Verification items for the finished model (mm, model axes). A direction names the side the tool comes from. Give positions to 0.01 mm unless a question says otherwise; leave off trailing zeros. Write each loop counter-clockwise with the first axis right and the second up, starting at its lowest first coordinate (ties: lowest second). Pieces come first, ordered by that corner, then holes. Notation, with made-up numbers: (-4.75, 16) - (8.25, 16) arc R26 cw to (8.25, 44) - close; hole circle Ø8 at (21, 29). An arc over 180 degrees is marked (long way). Answer as a JSON object with one key per item and string values. Group by question number.
Item 1: Sectioned sample at C-C, the plane x = -3.5. Record the boundary of the cut face in (y, z), and give its area (3 significant figures).
Item 2: Sectioned sample at B-B, the plane x = -27. Record the boundary of the cut face in (y, z).
Item 3: Sectioned sample at A-A, the plane y = 53.5. Record the boundary of the cut face in (x, z), and give its area (3 significant figures).
Item 4: Tool access check on faces 1 (the face through (-45.11, 2, 3)), 2 (the face through (-40.462, 6, 3)), 3 (the face through (-14, 0, 3)). Record the directions out of +Z, -Z, +X, -X, +Y, -Y that give a thin tool (end or side, any length) a straight path to the whole face; none if there is none.
Item 5: Scan lines: line 1 along X through (y, z) = (8.5, 1.6); line 2 along Y through (x, z) = (-34, 0.6); line 3 along Y through (x, z) = (-21, 4.4). Record each from-to range of solid material in increasing order. Write a range as [from, to].
Item 6: Go/stop test with flat-tipped pins: pin 1 (1.4 mm diameter, centred on x = -41, z = 3, fed in from -Y); pin 2 (0.9 mm diameter, centred on x = -43.5, z = 3.5, fed in from -Y) (3 decimals). Record where each tip stops, or that it passes through.
Item 7: Draft check along Y on faces 4 (the face through (-25, 19.467, 3)), 5 (the face through (-14, 49, 0)), 6 (the face through (-3, 0, 3)). Enter one of: +Y half, -Y half, draft (parallel to the pull), parting line (faces both ways), or undercut.
```python
from build123d import *

# Parameters (mm, degrees)
BOSS_EXTRUDE1_DEPTH = 5.9436
CUT_EXTRUDE1_DEPTH  = 6.9436
CUT_EXTRUDE2_DEPTH  = 6.9436


with BuildPart() as part:
    # Sketch2 → Boss-Extrude1 (new body)
    with BuildSketch(Plane.XY):
        Polygon((0, 0), (0, 101.6), (-50.8, 101.6), (-50.8, 0), (-31.75, 0), (-31.75, -5.9436), (-19.05, -5.9436), (-19.05, 0), align=None)
    extrude(amount=BOSS_EXTRUDE1_DEPTH)

    # Sketch3 → Cut-Extrude1 (cut, through all)
    with BuildSketch(Plane.XY.offset(5.9436)):
        Polygon((-27.965479444, 66.110608141), (-22.834520556, 66.110608141), (-21.792739864, 60.799784967), (-15.013102806, 60.799784967), (-15.013102806, 19.467361344), (-35.786897194, 19.467361344), (-35.786897194, 60.799784967), (-29.045829513, 60.8), align=None)
    extrude(amount=-CUT_EXTRUDE1_DEPTH, mode=Mode.SUBTRACT)

    # Sketch4 → Cut-Extrude2 (cut, through all)
    with BuildSketch(Plane.XY.offset(5.9436)):
        Polygon((-9.550241905, -0.00026), (-9.550241905, 4.60375), (-11.252041905, 4.60375), (-11.252041905, 6.985), (-9.550241905, 6.985), (-9.550241905, 9.525), (-6.603841905, 9.525), (-6.603841905, 6.985), (-4.902041905, 6.985), (-4.902041905, 4.60375), (-6.603841905, 4.60375), (-6.603841905, -0.00026), align=None)
        Polygon((-46.812041905, 4.60375), (-45.110241905, 4.60375), (-45.110241905, -0.00026), (-42.163841905, -0.00026), (-42.163841905, 4.60375), (-40.462041905, 4.60375), (-40.462041905, 6.985), (-42.163841905, 6.985), (-42.163841905, 9.525), (-45.110241905, 9.525), (-45.110241905, 6.985), (-46.812041905, 6.985), align=None)
    extrude(amount=-CUT_EXTRUDE2_DEPTH, mode=Mode.SUBTRACT)


solid = part.part
```
Geometry check:
{
 "1": {"outline": "(0, 0) - (101.6, 0) - (101.6, 5.94) - (0, 5.94) - close", "area": "604 mm^2"},
 "2": {"outline": "(-5.94, 0) - (19.47, 0) - (19.47, 5.94) - (-5.94, 5.94) - close; (66.11, 0) - (101.6, 0) - (101.6, 5.94) - (66.11, 5.94) - close"},
 "3": {"outline": "(-50.8, 0) - (-35.79, 0) - (-35.79, 5.94) - (-50.8, 5.94) - close; (-15.01, 0) - (0, 0) - (0, 5.94) - (-15.01, 5.94) - close", "area": "178 mm^2"},
 "4": {"face 1": "+Z, -Z, -Y", "face 2": "+Z, -Z", "face 3": "+Z, -Z, +X, -Y"},
 "5": {"line 1": "[-50.8, -45.11], [-42.16, -9.55], [-6.6, 0]", "line 2": "[0, 19.47], [60.8, 101.6]", "line 3": "[-5.94, 19.47], [60.8, 101.6]"},
 "6": {"pin 1": "y = 0", "pin 2": "y = 9.525"},
 "7": {"face 4": "undercut", "face 5": "draft", "face 6": "-Y half"}
}
